Can you work these out from the model? Positions are in its coordinate system, mm. A direction names the side the tool comes from. Give positions to 0.01 mm unless a question says otherwise; leave off trailing zeros. Loops run counter-clockwise (first coordinate to the right, second up) from the corner with the lowest first, then second, coordinate; pieces in that order, holes last. Notation, with made-up numbers: (32.25, 55) -> (67.25, 55) arc R23 ccw to (67.25, 68) -> close; hole circle Ø7 at (72, 30). An arc over 180 degrees is marked (long way). Return JSON: item names as keys, results as strings. Group by question number.
Q1. Suppose I cut it at A-A, the plane y = -18.5. Please give me the cut outline in (x, z).
Q2. Thinking about a two-plate mould opening in X: for faces 3 (the cylindrical face through (-2.352, -20.963, -3.944)), 4 (the flat face through (48.87, 14.75, -3.94)), 5 (the cylindrical face through (-24.705, -35.977, -3.944)), 6 (the flat face through (10, -38.727, -4)), which applies, pulls with the +X half, pulls with the -X half, needs draft (parallel to the pull), parting line crosses it, or undercut?
Q3. Suppose I cut it at C-C, the plane x = 11.5. Please give me the cut outline in (y, z).
Q4. Suppose I cut it at D-D, the plane y = -9. Please give me the cut outline in (x, z).
Q5. Suppose I cut it at B-B, the plane z = -2.75. Please give me the cut outline in (x, y).
Q6. Which directions (+Z, -Z, +X, -X, +Y, -Y) give clear straight access to the entire face, cutting with the end or side of a thin tool? Please do faces 1 (the flat face through (10, 16.273, -4)), 2 (the flat face through (43.095, -11, -4)).
Q7. I need wall thicknesses on line 1 along X through (y, z) = (8, -5.25); line 2 along X through (y, z) = (-30, -2); line 3 along X through (y, z) = (-15.5, -0.5). Which ranges of each line are inside material? Lowest first, please. Write a range as [from, to].
```python
from build123d import *

# Parameters (mm, degrees)
SKETCH1_W           = 80
SKETCH1_H           = 55
SKETCH1_R           = 16
BOSS_EXTRUDE1_DEPTH = 8
SKETCH2_R           = 2.25
CUT_EXTRUDE1_DEPTH  = 8
CIRPATTERN1_COUNT   = 3
CHAMFER1_SIZE       = 3


with BuildPart() as part:
    # Sketch1 → Boss-Extrude1 (new body)
    with BuildSketch(Plane.XY):
        with Locations((10.344708022, -11.227107004)):
            Rectangle(SKETCH1_W, SKETCH1_H)
        with Locations((10.344708022, -11.227107004)):
            Circle(SKETCH1_R, mode=Mode.SUBTRACT)
        with BuildLine():
            Line((-26.905291978, 11.272892996), (-26.905291978, -33.727107004))
            ThreePointArc((-26.905291978, -33.727107004), (-24.655291978, -35.977107004), (-22.405291978, -33.727107004))
            Line((-22.405291978, -33.727107004), (-22.405291978, 11.272892996))
            ThreePointArc((-22.405291978, 11.272892996), (-24.655291978, 13.522892996), (-26.905291978, 11.272892996))
        make_face(mode=Mode.SUBTRACT)
        with BuildLine():
            Line((43.094708022, 11.272892996), (43.094708022, -33.727107004))
            ThreePointArc((43.094708022, -33.727107004), (45.344708022, -35.977107004), (47.594708022, -33.727107004))
            Line((47.594708022, -33.727107004), (47.594708022, 11.272892996))
            ThreePointArc((47.594708022, 11.272892996), (45.344708022, 13.522892996), (43.094708022, 11.272892996))
        make_face(mode=Mode.SUBTRACT)
    extrude(amount=-BOSS_EXTRUDE1_DEPTH)

    # Sketch2 → Cut-Extrude1 (cut)
    with BuildSketch(Plane.XY):
        with Locations((10.344708022, -31.227107004)):
            Circle(SKETCH2_R)
    cut_extrude1 = extrude(amount=-CUT_EXTRUDE1_DEPTH, mode=Mode.SUBTRACT)

    # CirPattern1: Cut-Extrude1 ×3 about axis
    cirpattern1_axis = Axis((10.344708022, -11.227107004, 0), (0, 0, 1))
    for i in range(1, CIRPATTERN1_COUNT):
        add(cut_extrude1.rotate(cirpattern1_axis, i * 360 / CIRPATTERN1_COUNT), mode=Mode.SUBTRACT)

    # Chamfer1
    chamfer1_edges = [part.edges().sort_by_distance(p)[0] for p in [
        (-29.655291978, 16.272892996, -4),
        (50.344708022, 16.272892996, -4),
        (50.344708022, -38.727107004, -4),
        (-29.655291978, -38.727107004, -4),
    ]]
    chamfer(chamfer1_edges, length=CHAMFER1_SIZE)


solid = part.part
```
Ans:
{
 "1": {"outline": "(-29.66, -8) -> (-26.91, -8) -> (-26.91, 0) -> (-29.66, 0) -> close; (-22.41, -8) -> (-3.91, -8) -> (-3.91, 0) -> (-22.41, 0) -> close; (24.6, -8) -> (43.09, -8) -> (43.09, 0) -> (24.6, 0) -> close; (47.59, -8) -> (50.34, -8) -> (50.34, 0) -> (47.59, 0) -> close"},
 "2": {"face 3": "undercut", "face 4": "pulls with the +X half", "face 5": "undercut", "face 6": "needs draft"},
 "3": {"outline": "(-38.73, -8) -> (-33.16, -8) -> (-33.16, 0) -> (-38.73, 0) -> close; (-29.3, -8) -> (-27.19, -8) -> (-27.19, 0) -> (-29.3, 0) -> close; (4.73, -8) -> (16.27, -8) -> (16.27, 0) -> (4.73, 0) -> close"},
 "4": {"outline": "(-29.66, -8) -> (-26.91, -8) -> (-26.91, 0) -> (-29.66, 0) -> close; (-22.41, -8) -> (-5.5, -8) -> (-5.5, 0) -> (-22.41, 0) -> close; (26.19, -8) -> (43.09, -8) -> (43.09, 0) -> (26.19, 0) -> close; (47.59, -8) -> (50.34, -8) -> (50.34, 0) -> (47.59, 0) -> close"},
 "5": {"outline": "(-29.66, -35.73) -> (-26.66, -38.73) -> (47.34, -38.73) -> (50.34, -35.73) -> (50.34, 13.27) -> (47.34, 16.27) -> (-26.66, 16.27) -> (-29.66, 13.27) -> close; hole (-26.91, -33.73) arc R2.25 ccw to (-22.41, -33.73) -> (-22.41, 11.27) arc R2.25 ccw to (-26.91, 11.27) -> close; hole circle Ø4.5 at (-6.98, -1.23); hole circle Ø32 at (10.34, -11.23); hole circle Ø4.5 at (10.34, -31.23); hole circle Ø4.5 at (27.67, -1.23); hole (43.09, -33.73) arc R2.25 ccw to (47.59, -33.73) -> (47.59, 11.27) arc R2.25 ccw to (43.09, 11.27) -> close"},
 "6": {"face 1": "+Z, -Z, +X, -X, +Y", "face 2": "+Z, -Z"},
 "7": {"line 1": "x = [-29.66, -26.91], [-22.41, 43.09], [47.59, 50.34]", "line 2": "x = [-29.66, -26.91], [-22.41, 8.46], [12.23, 43.09], [47.59, 50.34]", "line 3": "x = [-29.66, -26.91], [-22.41, -5.07], [25.76, 43.09], [47.59, 50.34]"}
}
